```python
from build123d import *

# Parameters (mm, degrees)
F0_W     = 60
F0_H     = 115
F1_DEPTH = 20
F3_W     = 55.999996
F3_H     = 110.999996
F4_DEPTH = 9
F2_W     = 55
F2_H     = 8
F5_DEPTH = 114
F6_R     = 1.25
F7_DEPTH = 1
F8_SIZE  = 1


with BuildPart() as f1:
    # F0 (on Front) → F1 (new body)
    with BuildSketch(Plane.XZ):
        with Locations((30, 57.5)):
            Rectangle(F0_W, F0_H)
    extrude(amount=F1_DEPTH)

    # F3 (on face) → F4 (cut)
    with BuildSketch(Plane(origin=(0, 0, 0), x_dir=(-1, 0, 0), z_dir=(0, 1, 0))):
        with Locations((-30, 57.5)):
            Rectangle(F3_W, F3_H)
    extrude(amount=-F4_DEPTH, mode=Mode.SUBTRACT)

    # F2 (on face) → F5 (cut)
    with BuildSketch(Plane.XY.offset(115)):
        with Locations((30, -15)):
            Rectangle(F2_W, F2_H)
    extrude(amount=-F5_DEPTH, mode=Mode.SUBTRACT)

    # F6 (on face) → F7 (cut)
    with BuildSketch(Plane.XZ.offset(20)):
        with BuildLine():
            Line((28.75, 26), (28.75, 9.5))
            ThreePointArc((28.75, 9.5), (30, 8.25), (31.25, 9.5))
            Line((31.25, 9.5), (31.25, 26))
            ThreePointArc((31.25, 26), (30, 27.25), (28.75, 26))
        make_face()
        with Locations((30, 6)):
            Circle(F6_R)
    extrude(amount=-F7_DEPTH, mode=Mode.SUBTRACT)

    # F8
    f8_edges = [f1.edges().sort_by_distance(p)[0] for p in [
        (0, -20, 57.5),
        (60, -20, 57.5),
        (30, -20, 0),
        (60, -10, 0),
        (30, 0, 0),
        (0, -10, 0),
        (0, 0, 57.5),
        (60, 0, 57.5),
    ]]
    chamfer(f8_edges, length=F8_SIZE)


solid = f1.part
```
Verification items for the finished model (mm, model axes). A direction names the side the tool comes from. Give positions to 0.01 mm unless a question says otherwise; leave off trailing zeros. Order: outer loops, then holes, each group sorted by start corner. A loop starts at its lowest first (then second) coordinate and runs counter-clockwise, first axis right, second up. Notation, with made-up numbers: M 85.5,3.5 L 130.5,3.5 A18 ccw 130.5,22.5 Z; hole C 30,-21 d4. An arc over 180 degrees is marked long. Return JSON: item names as keys, results as strings. Group by question number.
1) Go/stop test with flat-tipped pins: pin 1 Ø0.5 at (y, z) = (-19.5, 21) entering from +X; pin 2 Ø1 at (x, z) = (14, 21) entering from +Y; pin 3 Ø2 at (x, z) = (30, 6) entering from -Y. Record where each tip stops, or that it passes through.
2) Section check C-C on y = -7.5. Record the cut outline in (x, z), and give its area (3 significant figures).
3) Section check D-D on x = 22. Record the cut outline in (y, z).
4) Section check B-B on z = 68.5. Record the cut outline in (x, y).
5) Mould release check, pull along X, two halves, no side actions. Record for faces 1 (the face through (0, -10, 57)), 2 (the face through (2, -4, 57)), 3 (the face through (30, -20, 59)): pulls with the +X half, pulls with the -X half, needs draft (parallel to the pull), parting line crosses it, or undercut.
6) Section check A-A on x = 30. Record the cut outline in (y, z).
7) Scan lines: line 1 (X direction, y = -12, z = 31); line 2 (Y direction, x = 11, z = 47); line 3 (Z direction, x = 30, y = -19.2). Record each from-to range of solid material in increasing order.
8) Access from +Z, -Z, +X, -X, +Y, -Y to the whole of each face (thin tool, end or side, straight path). Record for faces 4 (the face through (2.5, -15, 59)), 5 (the face through (30, -4, 113)), 6 (the face through (30.577, -19.507, 4.891)), 7 (the face through (30, -10, 0)).
Answer block:
{
 "1": {"pin 1": "stops at x = 59.75", "pin 2": "stops at y = -9", "pin 3": "stops at y = -11"},
 "2": {"outline": "M 0,1 L 1,0 L 59,0 L 60,1 L 60,115 L 0,115 Z; hole M 2,2 L 58,2 L 58,113 L 2,113 Z", "area": "683 mm^2"},
 "3": {"outline": "M -20,1 L -19,0 L -1,0 L 0,1 L 0,2 L -9,2 L -9,113 L 0,113 L 0,115 L -11,115 L -11,1 L -19,1 L -19,115 L -20,115 Z"},
 "4": {"outline": "M 0,-19 L 1,-20 L 59,-20 L 60,-19 L 60,-1 L 59,0 L 58,0 L 58,-9 L 2,-9 L 2,0 L 1,0 L 0,-1 Z; hole M 2.5,-19 L 57.5,-19 L 57.5,-11 L 2.5,-11 Z"},
 "5": {"face 1": "pulls with the -X half", "face 2": "undercut", "face 3": "needs draft"},
 "6": {"outline": "M -20,1 L -19,0 L -1,0 L 0,1 L 0,2 L -9,2 L -9,113 L 0,113 L 0,115 L -11,115 L -11,1 L -19,1 L -19,4.75 L -20,4.75 Z; M -20,7.25 L -19,7.25 L -19,8.25 L -20,8.25 Z; M -20,27.25 L -19,27.25 L -19,115 L -20,115 Z"},
 "7": {"line 1": "x = 0 to 2.5, 57.5 to 60", "line 2": "y = -20 to -19, -11 to -9", "line 3": "z = 0.2 to 4.75, 7.25 to 8.25, 27.25 to 115"},
 "8": {"face 4": "+Z", "face 5": "+Y", "face 6": "-Y", "face 7": "-Z, +X, -X, +Y, -Y"}
}
